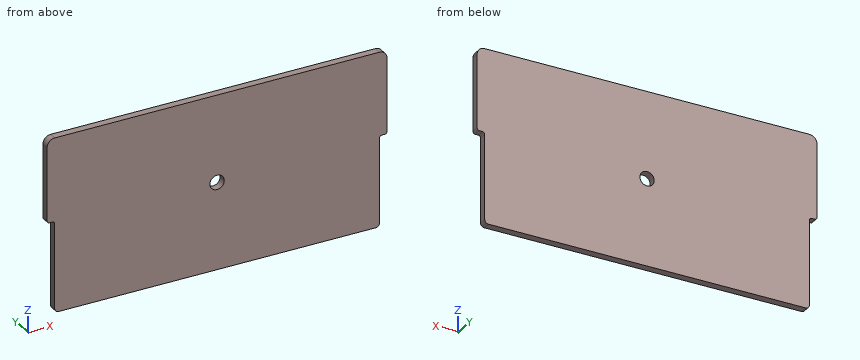
```python
from build123d import *

# Parameters (mm, degrees)
SKETCH2_W           = 450
SKETCH2_H           = 230
BOSS_EXTRUDE2_DEPTH = 10
SKETCH4_W           = 10
SKETCH4_H           = 120
CUT_EXTRUDE2_DEPTH  = 286
FILLET1_R           = 10
FILLET7_R           = 3
FILLET8_R           = 5
FILLET9_R           = 3
FILLET10_R          = 10
SKETCH5_R           = 9.5
CUT_EXTRUDE4_DEPTH  = 10


with BuildPart() as part:
    # Sketch2 → Boss-Extrude2 (new body)
    with BuildSketch(Plane(origin=(0, 0, 0), x_dir=(1, 0, 0), z_dir=(0, 1, 0))):
        with Locations((176.829853391, -84.071504635)):
            Rectangle(SKETCH2_W, SKETCH2_H)
    extrude(amount=BOSS_EXTRUDE2_DEPTH)

    # Sketch4 → Cut-Extrude2 (cut)
    with BuildSketch(Plane(origin=(0, 10, 0), x_dir=(1, 0, 0), z_dir=(0, 1, 0))):
        with Locations((-43.170146609, -29.071504635)):
            Rectangle(SKETCH4_W, SKETCH4_H)
        with Locations((396.829853391, -29.071504635)):
            Rectangle(SKETCH4_W, SKETCH4_H)
    extrude(amount=-CUT_EXTRUDE2_DEPTH, mode=Mode.SUBTRACT)

    # Fillet1
    fillet1_edges = [part.edges().sort_by_distance(p)[0] for p in [
        (-48.170146609, 5, 199.071504635),
    ]]
    fillet(fillet1_edges, radius=FILLET1_R)

    # Fillet7
    fillet7_edges = [part.edges().sort_by_distance(p)[0] for p in [
        (-48.170146609, 5, 89.071504635),
        (-38.170146609, 5, 89.071504635),
    ]]
    fillet(fillet7_edges, radius=FILLET7_R)

    # Fillet8
    fillet8_edges = [part.edges().sort_by_distance(p)[0] for p in [
        (-38.170146609, 5, -30.928495365),
        (391.829853391, 5, -30.928495365),
    ]]
    fillet(fillet8_edges, radius=FILLET8_R)

    # Fillet9
    fillet9_edges = [part.edges().sort_by_distance(p)[0] for p in [
        (401.829853391, 5, 89.071504635),
        (391.829853391, 5, 89.071504635),
    ]]
    fillet(fillet9_edges, radius=FILLET9_R)

    # Fillet10
    fillet10_edges = [part.edges().sort_by_distance(p)[0] for p in [
        (401.829853391, 5, 199.071504635),
    ]]
    fillet(fillet10_edges, radius=FILLET10_R)

    # Sketch5 → Cut-Extrude4 (cut)
    with BuildSketch(Plane(origin=(0, 10, 0), x_dir=(1, 0, 0), z_dir=(0, 1, 0))):
        with Locations(Location((176.829853391, -84.071504635, 0), (0, 0, 270))):
            Circle(SKETCH5_R)
    extrude(amount=-CUT_EXTRUDE4_DEPTH, mode=Mode.SUBTRACT)


solid = part.part
```
The listing builds one solid part. Answer for the finished solid, in the listing's coordinates (mm). Round coordinates to 2 decimals unless told otherwise and drop trailing zeros. Order: outer loops, then holes, each group sorted by start corner. A loop starts at its lowest first (then second) coordinate and runs counter-clockwise, first axis right, second up. Notation, with made-up numbers: (63.5, 16.5) -> (122.5, 16.5) arc R14 ccw to (122.5, 21.5) -> close; hole circle Ø2 at (59, 54). An arc over 180 degrees is marked (long way). Answer as CSV lines item,"result". Start each with the question number.
(1) Flat-ended cylindrical pins translate along their axes: pin 1 Ø3 at (x, y) = (397.5, 4.5) entering from -Z; pin 2 Ø17 at (x, z) = (176.83, 84.07) entering from -Y. Find the tip coordinate at first contact, or state that the pin passes through.
(2) Find the intervals of material crossed by probe 1 along X at (y, z) = (6.25, 5.5); probe 2 along X at (y, z) = (1.5, 77); probe 3 along Z at (x, y) = (184.5, 6.5), in increasing order. Write a range as from..to.
(3) The part is cut by section A-A (y = 5.75). Determine the outline of the cut face in (x, z), then the cut area to 3 significant figures.
(4) The part is cut by section B-B (z = 47). Determine the outline of the cut face in (x, y).
Evaluation:
1,pin 1,"z = 89.07"
1,pin 2,"through"
2,probe 1,"-38.17..391.83"
2,probe 2,"-38.17..170.49, 183.17..391.83"
2,probe 3,"-30.93..78.47, 89.68..199.07"
3,outline,"(-48.17, 92.07) arc R3 ccw to (-45.17, 89.07) -> (-41.17, 89.07) arc R3 cw to (-38.17, 86.07) -> (-38.17, -25.93) arc R5 ccw to (-33.17, -30.93) -> (386.83, -30.93) arc R5 ccw to (391.83, -25.93) -> (391.83, 86.07) arc R3 cw to (394.83, 89.07) -> (398.83, 89.07) arc R3 ccw to (401.83, 92.07) -> (401.83, 189.07) arc R10 ccw to (391.83, 199.07) -> (-38.17, 199.07) arc R10 ccw to (-48.17, 189.07) -> close; hole circle Ø19 at (176.83, 84.07)"
3,area,"101,000 mm²"
4,outline,"(-38.17, 0) -> (391.83, 0) -> (391.83, 10) -> (-38.17, 10) -> close"
